Read the model definition and answer for the solid it produces. Units are mm, in the model's axes. Face numbers are marked on the shaded views. Round coordinates to 2 decimals unless told otherwise and drop trailing zeros. Write each loop counter-clockwise with the first axis right and the second up, starting at its lowest first coordinate (ties: lowest second). Pieces come first, ordered by that corner, then holes. Notation, with made-up numbers: (-0.75, 15) - (56.25, 15) arc R31 ccw to (56.25, 47) - close; hole circle Ø11 at (-3, 71.25). An arc over 180 degrees is marked (long way). One line per item, written item: value. Start each with the question number.
(1) The mould has two halves that part along Z. Classify the marked faces 1, 2, 3 and 4: +Z half, -Z half, draft (parallel to the pull), parting line (faces both ways), or undercut.
(2) A cutting plane is placed at C-C, the plane z = -7.5. Determine the outline of the cut face in (x, y).
(3) A cutting plane is placed at D-D, the plane y = -96. Determine the outline of the cut face in (x, z), plus the area to 3 significant figures.
(4) Find the intervals of material crossed by L1, parallel to X at y = -234, z = -2; L2, parallel to Z at x = -29, y = -39.5; L3, parallel to X at y = -16, z = -66, in increasing order.
(5) A cutting plane is placed at B-B, the plane x = 11.5. Determine the outline of the cut face in (y, z), plus the area to 3 significant figures.
(6) A cutting plane is placed at A-A, the plane y = -233. Determine the outline of the cut face in (x, z), plus the area to 3 significant figures.
(7) Flat-ended cylindrical pins translate along their axes: pin 1 Ø11.5 at (x, z) = (-25.5, -20) entering from +Y; pin 2 Ø4 at (y, z) = (-74, 34) entering from -X; pin 3 Ø5 at (x, z) = (-52, 60.5) entering from -Y; pin 4 Ø6 at (x, y) = (-47.5, -113) entering from +Z. Find the tip coordinate at first contact, or state that the pin passes through.
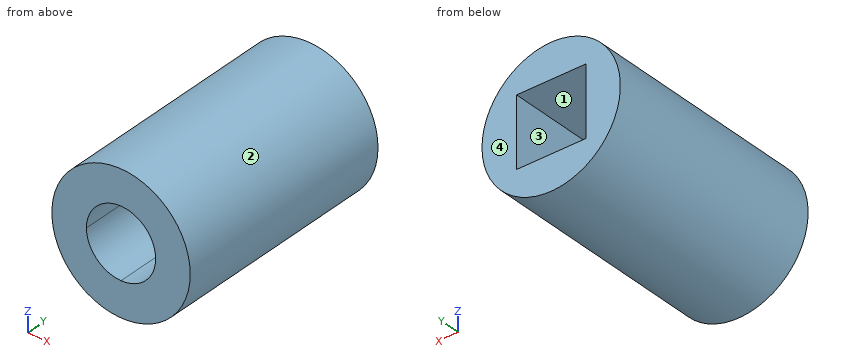
from build123d import *

# Parameters (mm, degrees)
F0_R     = 76.2
F2_DEPTH = 254
F3_DEPTH = 254.001
F4_DEPTH = 101.6


with BuildPart() as f2:
    # F0 (on Front) → F2 (new body)
    with BuildSketch(Plane.XZ):
        Circle(F0_R)
    extrude(amount=F2_DEPTH)

    # F1 (on Front) → F3 (cut, through all)
    with BuildSketch(Plane.XZ):
        with BuildLine():
            ThreePointArc((38.1, 0), (26.940768, 26.940768), (0, 38.1))
            ThreePointArc((0, 38.1), (-26.940768, 26.940768), (-38.1, 0))
            ThreePointArc((-38.1, 0), (-26.940768, -26.940768), (0, -38.1))
            ThreePointArc((0, -38.1), (26.940768, -26.940768), (38.1, 0))
        make_face()
    extrude(amount=F3_DEPTH, mode=Mode.SUBTRACT)

    # F1 (on Front) → F4 (cut)
    with BuildSketch(Plane.XZ):
        with BuildLine():
            Line((38.1, 0), (38.1, 38.1))
            Line((38.1, 38.1), (0, 38.1))
            ThreePointArc((0, 38.1), (26.940768, 26.940768), (38.1, 0))
        make_face()
        with BuildLine():
            ThreePointArc((-38.1, 0), (-26.940768, 26.940768), (0, 38.1))
            Line((0, 38.1), (-38.1, 38.1))
            Line((-38.1, 38.1), (-38.1, 0))
        make_face()
        with BuildLine():
            Line((38.1, -38.1), (38.1, 0))
            ThreePointArc((38.1, 0), (26.940768, -26.940768), (0, -38.1))
            Line((0, -38.1), (38.1, -38.1))
        make_face()
        with BuildLine():
            ThreePointArc((0, -38.1), (-26.940768, -26.940768), (-38.1, 0))
            Line((-38.1, 0), (-38.1, -38.1))
            Line((-38.1, -38.1), (0, -38.1))
        make_face()
    extrude(amount=F4_DEPTH, mode=Mode.SUBTRACT)


solid = f2.part
Here are the results:
1. face 1: undercut
1. face 2: parting line
1. face 3: undercut
1. face 4: draft
2. outline: (-75.83, -254) - (-37.35, -254) - (-37.35, -101.6) - (-38.1, -101.6) - (-38.1, 0) - (-75.83, 0) - close; (37.35, -254) - (75.83, -254) - (75.83, 0) - (38.1, 0) - (38.1, -101.6) - (37.35, -101.6) - close
3. outline: circle Ø152.4 at (0, 0); hole (-38.1, -38.1) - (38.1, -38.1) - (38.1, 38.1) - (-38.1, 38.1) - close
3. area: 12,400 mm²
4. L1: -76.17 to -38.05, 38.05 to 76.17
4. L2: -70.47 to -38.1, 38.1 to 70.47
4. L3: -38.08 to 38.08
5. outline: (-254, -75.33) - (0, -75.33) - (0, -38.1) - (-101.6, -38.1) - (-101.6, -36.32) - (-254, -36.32) - close; (-254, 36.32) - (-101.6, 36.32) - (-101.6, 38.1) - (0, 38.1) - (0, 75.33) - (-254, 75.33) - close
5. area: 19,500 mm²
6. outline: circle Ø152.4 at (0, 0); hole (-38.1, 0) arc R38.1 ccw to (0, -38.1) arc R38.1 ccw to (38.1, 0) arc R38.1 ccw to (0, 38.1) arc R38.1 ccw to start
6. area: 13,700 mm²
7. pin 1: y = -101.6
7. pin 2: x = -69.16
7. pin 3: through
7. pin 4: z = 61.86
